```python
from build123d import *

# Parameters (mm, degrees)
SKETCH1_W           = 304.8
SKETCH1_H           = 304.8
SKETCH1_W_2         = 93
SKETCH1_H_2         = 93
BOSS_EXTRUDE1_DEPTH = 15.24
SKETCH2_W           = 304.8
SKETCH2_H           = 304.8
BOSS_EXTRUDE2_DEPTH = 3.175
SKETCH3_W           = 304.8
SKETCH3_H           = 304.8
SKETCH3_W_2         = 254
SKETCH3_H_2         = 254
BOSS_EXTRUDE3_DEPTH = 10
SKETCH4_OUTSIDE_W   = 393.198
SKETCH4_OUTSIDE_H   = 393.198
SKETCH4_OUTSIDE_W_2 = 260.35
SKETCH4_OUTSIDE_H_2 = 260.35
CUT_EXTRUDE1_DEPTH  = 25.24
SKETCH5_R           = 3.4925
CUT_EXTRUDE2_DEPTH  = 217.999026726
SKETCH6_W           = 25.4
SKETCH6_H           = 6.35
CUT_EXTRUDE3_DEPTH  = 15.24
SKETCH7_W           = 388.208697242
SKETCH7_H           = 185.968986832
CUT_EXTRUDE4_DEPTH  = 323.042618647
SKETCH8_W           = 545.051384684
SKETCH8_H           = 463.265958
CUT_EXTRUDE5_DEPTH  = 323.042618647
SKETCH9_W           = 585.539242267
SKETCH9_H           = 383.639310532
CUT_EXTRUDE6_DEPTH  = 303.729153039


with BuildPart() as part:
    # Sketch1 → Boss-Extrude1 (new body)
    with BuildSketch(Plane(origin=(0, 0, 0), x_dir=(1, 0, 0), z_dir=(0, 1, 0))):
        Rectangle(SKETCH1_W, SKETCH1_H)
        with Locations((58.057, 58.057)):
            Rectangle(SKETCH1_W_2, SKETCH1_H_2, mode=Mode.SUBTRACT)
        with Locations((-58.057, 58.057)):
            Rectangle(SKETCH1_W_2, SKETCH1_H_2, mode=Mode.SUBTRACT)
        with Locations((-58.057, -58.057)):
            Rectangle(SKETCH1_W_2, SKETCH1_H_2, mode=Mode.SUBTRACT)
        with Locations((58.057, -58.057)):
            Rectangle(SKETCH1_W_2, SKETCH1_H_2, mode=Mode.SUBTRACT)
    extrude(amount=BOSS_EXTRUDE1_DEPTH)

    # Sketch2 → Boss-Extrude2 (add)
    with BuildSketch(Plane(origin=(0, 0, 0), x_dir=(-1, 0, 0), z_dir=(0, -1, 0))):
        Rectangle(SKETCH2_W, SKETCH2_H)
    extrude(amount=BOSS_EXTRUDE2_DEPTH)

    # Sketch3 → Boss-Extrude3 (add)
    with BuildSketch(Plane(origin=(0, 15.24, 0), x_dir=(1, 0, 0), z_dir=(0, 1, 0))):
        Rectangle(SKETCH3_W, SKETCH3_H)
        Rectangle(SKETCH3_W_2, SKETCH3_H_2, mode=Mode.SUBTRACT)
    extrude(amount=BOSS_EXTRUDE3_DEPTH)

    # Sketch4 outside → Cut-Extrude1 (cut)
    with BuildSketch(Plane(origin=(0, 25.24, 0), x_dir=(1, 0, 0), z_dir=(0, 1, 0))):
        Rectangle(SKETCH4_OUTSIDE_W, SKETCH4_OUTSIDE_H)
        Rectangle(SKETCH4_OUTSIDE_W_2, SKETCH4_OUTSIDE_H_2, mode=Mode.SUBTRACT)
    extrude(amount=-CUT_EXTRUDE1_DEPTH, mode=Mode.SUBTRACT)

    # Sketch5 → Cut-Extrude2 (cut, through all)
    with BuildSketch(Plane(origin=(0, 0, 0), x_dir=(1, 0, 0), z_dir=(0, 1, 0))):
        with Locations(Location((-139.7, -139.7, 0), (0, 0, 270))):
            Circle(SKETCH5_R)
        with Locations(Location((-114.3, -139.7, 0), (0, 0, 270))):
            Circle(SKETCH5_R)
        with Locations(Location((-88.9, -139.7, 0), (0, 0, 270))):
            Circle(SKETCH5_R)
        with Locations(Location((-63.5, -139.7, 0), (0, 0, 270))):
            Circle(SKETCH5_R)
        with Locations(Location((-38.1, -139.7, 0), (0, 0, 270))):
            Circle(SKETCH5_R)
        with Locations(Location((-12.7, -139.7, 0), (0, 0, 270))):
            Circle(SKETCH5_R)
        with Locations(Location((12.7, -139.7, 0), (0, 0, 270))):
            Circle(SKETCH5_R)
        with Locations(Location((38.1, -139.7, 0), (0, 0, 270))):
            Circle(SKETCH5_R)
        with Locations(Location((63.5, -139.7, 0), (0, 0, 270))):
            Circle(SKETCH5_R)
        with Locations(Location((88.9, -139.7, 0), (0, 0, 270))):
            Circle(SKETCH5_R)
        with Locations(Location((114.3, -139.7, 0), (0, 0, 270))):
            Circle(SKETCH5_R)
        with Locations(Location((139.7, -139.7, 0), (0, 0, 270))):
            Circle(SKETCH5_R)
        with Locations(Location((-139.7, -114.3, 0), (0, 0, 270))):
            Circle(SKETCH5_R)
        with Locations(Location((-139.7, -88.9, 0), (0, 0, 270))):
            Circle(SKETCH5_R)
        with Locations(Location((-139.7, -63.5, 0), (0, 0, 270))):
            Circle(SKETCH5_R)
        with Locations(Location((-139.7, -38.1, 0), (0, 0, 270))):
            Circle(SKETCH5_R)
        with Locations(Location((-139.7, -12.7, 0), (0, 0, 270))):
            Circle(SKETCH5_R)
        with Locations(Location((-139.7, 12.7, 0), (0, 0, 270))):
            Circle(SKETCH5_R)
        with Locations(Location((-139.7, 38.1, 0), (0, 0, 270))):
            Circle(SKETCH5_R)
        with Locations(Location((-139.7, 63.5, 0), (0, 0, 270))):
            Circle(SKETCH5_R)
        with Locations(Location((-139.7, 88.9, 0), (0, 0, 270))):
            Circle(SKETCH5_R)
        with Locations(Location((-139.7, 114.3, 0), (0, 0, 270))):
            Circle(SKETCH5_R)
        with Locations(Location((-139.7, 139.7, 0), (0, 0, 270))):
            Circle(SKETCH5_R)
        with Locations(Location((-114.3, 139.7, 0), (0, 0, 270))):
            Circle(SKETCH5_R)
        with Locations(Location((-88.9, 139.7, 0), (0, 0, 270))):
            Circle(SKETCH5_R)
        with Locations(Location((-63.5, 139.7, 0), (0, 0, 270))):
            Circle(SKETCH5_R)
        with Locations(Location((-38.1, 139.7, 0), (0, 0, 270))):
            Circle(SKETCH5_R)
        with Locations(Location((-12.7, 139.7, 0), (0, 0, 270))):
            Circle(SKETCH5_R)
        with Locations(Location((12.7, 139.7, 0), (0, 0, 270))):
            Circle(SKETCH5_R)
        with Locations(Location((38.1, 139.7, 0), (0, 0, 270))):
            Circle(SKETCH5_R)
        with Locations(Location((63.5, 139.7, 0), (0, 0, 270))):
            Circle(SKETCH5_R)
        with Locations(Location((88.9, 139.7, 0), (0, 0, 270))):
            Circle(SKETCH5_R)
        with Locations(Location((114.3, 139.7, 0), (0, 0, 270))):
            Circle(SKETCH5_R)
        with Locations(Location((139.7, 139.7, 0), (0, 0, 270))):
            Circle(SKETCH5_R)
        with Locations(Location((139.7, 114.3, 0), (0, 0, 270))):
            Circle(SKETCH5_R)
        with Locations(Location((139.7, 88.9, 0), (0, 0, 270))):
            Circle(SKETCH5_R)
        with Locations(Location((139.7, 63.5, 0), (0, 0, 270))):
            Circle(SKETCH5_R)
        with Locations(Location((139.7, 38.1, 0), (0, 0, 270))):
            Circle(SKETCH5_R)
        with Locations(Location((139.7, 12.7, 0), (0, 0, 270))):
            Circle(SKETCH5_R)
        with Locations(Location((139.7, -12.7, 0), (0, 0, 270))):
            Circle(SKETCH5_R)
        with Locations(Location((139.7, -38.1, 0), (0, 0, 270))):
            Circle(SKETCH5_R)
        with Locations(Location((139.7, -63.5, 0), (0, 0, 270))):
            Circle(SKETCH5_R)
        with Locations(Location((139.7, -88.9, 0), (0, 0, 270))):
            Circle(SKETCH5_R)
        with Locations(Location((139.7, -114.3, 0), (0, 0, 270))):
            Circle(SKETCH5_R)
    extrude(amount=-CUT_EXTRUDE2_DEPTH, mode=Mode.SUBTRACT)

    # Sketch6 → Cut-Extrude3 (cut)
    with BuildSketch(Plane(origin=(0, 15.24, 0), x_dir=(1, 0, 0), z_dir=(0, 1, 0))):
        with Locations((-58.057, 107.732)):
            Rectangle(SKETCH6_W, SKETCH6_H)
        with Locations((-58.057, -8.382)):
            Rectangle(SKETCH6_W, SKETCH6_H)
        with Locations((-58.057, 8.382)):
            Rectangle(SKETCH6_W, SKETCH6_H)
        with Locations((-58.057, -107.732)):
            Rectangle(SKETCH6_W, SKETCH6_H)
        with Locations((58.057, -107.732)):
            Rectangle(SKETCH6_W, SKETCH6_H)
        with Locations((58.057, -8.382)):
            Rectangle(SKETCH6_W, SKETCH6_H)
        with Locations((58.057, 8.382)):
            Rectangle(SKETCH6_W, SKETCH6_H)
        with Locations((58.057, 107.732)):
            Rectangle(SKETCH6_W, SKETCH6_H)
    extrude(amount=-CUT_EXTRUDE3_DEPTH, mode=Mode.SUBTRACT)

    # Sketch7 → Cut-Extrude4 (cut, through all)
    with BuildSketch(Plane(origin=(0, 0, -130.175), x_dir=(-1, 0, 0), z_dir=(0, 0, -1))):
        with Locations((-26.237813245, -25.540582214)):
            Rectangle(SKETCH7_W, SKETCH7_H)
    extrude(amount=CUT_EXTRUDE4_DEPTH, mode=Mode.SUBTRACT)

    # Sketch8 → Cut-Extrude5 (cut, through all)
    with BuildSketch(Plane.ZY.offset(130.175)):
        with Locations((35.238029092, 25.908608745)):
            Rectangle(SKETCH8_W, SKETCH8_H)
    extrude(amount=CUT_EXTRUDE5_DEPTH, mode=Mode.SUBTRACT)

    # Sketch9 → Cut-Extrude6 (cut, through all)
    with BuildSketch(Plane(origin=(130.175, 0, 0), x_dir=(0, 0, -1), z_dir=(1, 0, 0))):
        with Locations((26.844145207, 44.758305083)):
            Rectangle(SKETCH9_W, SKETCH9_H)
    extrude(amount=CUT_EXTRUDE6_DEPTH, mode=Mode.SUBTRACT)


solid = part.part
```
Read the model definition and answer for the solid it produces. Units are mm, in the model's axes. A direction names the side the tool comes from. Give positions to 0.01 mm unless a question says otherwise; leave off trailing zeros. Order: outer loops, then holes, each group sorted by start corner. A loop starts at its lowest first (then second) coordinate and runs counter-clockwise, first axis right, second up.
(1) Find section C-C (y = 20). Give the vertices of the cut face in (x, z) (3 decimals), plus the area to 3 significant figures.
(2) For a pull along Z with two mould halves and no side action, classify faces 3 (the flat face through (130.175, 11, 13)), 4 (the flat face through (-88, 8, -11.557)), 5 (the flat face through (2, 11, -130.175)) as released by +Z, released by -Z, zero draft, split by the parting line, or undercut.
(3) Straight lines are drawn through the part: L1, parallel to X at y = 3.5, z = 64.5 (3 decimals); L2, parallel to Z at x = 17, y = 18.5 (3 decimals). For each, find the intervals that lie inside material, in ascending order.
(4) For faces 1 (the flat face through (-70.757, 8, -108)), 2 (the cylindrical face through (-65.63, -1.57, 136.93)), determine the directions among +Z, -Z, +X, -X, +Y, -Y from which every point of the face is accessible in a straight line to the end or side of a thin tool.
(5) Find section D-D (x = -6). Give the vertices of the cut face in (y, z) (3 decimals).
(6) Find section A-A (x = 114.3). Give the vertices of the cut face in (y, z) (1 decimal), plus the area to 3 significant figures.
(7) Find section B-B (z = -82.5). Give the vertices of the cut face in (x, y) (3 decimals).
(8) Given pin 1 (17 mm diameter, centred on x = 34.5, y = 10, fed in from +Z) (3 decimals); pin 2 (8 mm diameter, centred on x = 114.3, z = 139.7, fed in from +Y); pin 3 (5.5 mm diameter, centred on x = -38.1, z = 139.7, fed in from +Y) (3 decimals), each flat-ended and moving along its own axis, determine where each tip first touches the part or whether it passes through.
Result sheet:
1. outline: (-130.175, -130.175) - (130.175, -130.175) - (130.175, 130.175) - (-130.175, 130.175) - close; hole (-127, -127) - (127, -127) - (127, 127) - (-127, 127) - close
1. area: 3,270 mm2
2. face 3: zero draft
2. face 4: undercut
2. face 5: released by -Z
3. L1: x = -130.175 to -104.557, -11.557 to 11.557, 104.557 to 130.175
3. L2: z = -130.175 to -127, 127 to 130.175
4. face 1: +Y
4. face 2: +Y, -Y
5. outline: (-3.175, -130.175) - (25.24, -130.175) - (25.24, -127) - (15.24, -127) - (15.24, 127) - (25.24, 127) - (25.24, 130.175) - (0, 130.175) - (0, 152.4) - (-3.175, 152.4) - close
6. outline: (-3.2, -130.2) - (25.2, -130.2) - (25.2, -127) - (15.2, -127) - (15.2, 127) - (25.2, 127) - (25.2, 130.2) - (0, 130.2) - (0, 136.2) - (-3.2, 136.2) - close; (-3.2, 143.2) - (0, 143.2) - (0, 152.4) - (-3.2, 152.4) - close
6. area: 4,910 mm2
7. outline: (-130.175, -3.175) - (130.175, -3.175) - (130.175, 25.24) - (127, 25.24) - (127, 15.24) - (104.557, 15.24) - (104.557, 0) - (11.557, 0) - (11.557, 15.24) - (-11.557, 15.24) - (-11.557, 0) - (-104.557, 0) - (-104.557, 15.24) - (-127, 15.24) - (-127, 25.24) - (-130.175, 25.24) - close
8. pin 1: stops at z = 130.175
8. pin 2: stops at y = 0
8. pin 3: passes through
